Solid Edge part; units mm, degrees
sketch "Sketch1" plane through (0, 0, 0) normal (0, -1, 0) x (1, 0, 0)
  line L0 (-30, 3.5) -> (30, 3.5)
  line L1 (30, 3.5) -> (30, -3.5)
  line L2 (30, -3.5) -> (-30, -3.5)
  line L3 (-30, -3.5) -> (-30, 3.5)
  dimension "D1" = 30
  dimension "D2" = 30
extrude "Protrusion1" add sketch "Sketch1" against normal blind 70
sketch "Sketch2" plane through (0, 35, 3.5) normal (0, 0, 1) x (0, 1, 0)
  line L0 (15, 3) -> (-15, 3)
  line L1 (-15, 3) -> (-15, -3)
  line L2 (-15, -3) -> (15, -3)
  line L3 (15, -3) -> (15, 3)
  dimension "D1" = 15
  dimension "D2" = 15
extrude "Utskärning_för_vertikal_pelare" cut sketch "Sketch2" against normal blind 5
fillet "Avrundningar_1" radius 1 8 edges at (-30, 35, 3.5) (0, 0, 3.5) (30, 35, 3.5) (0, 70, 3.5) (30, 70, 0) (30, 0, 0) (-30, 70, 0) (-30, 0, 0)
Can you work these out from the model? Positions are in its coordinate system, mm. A direction names the side the tool comes from. Round coordinates to 2 decimals unless told otherwise and drop trailing zeros. Order: outer loops, then holes, each group sorted by start corner. A loop starts at its lowest first (then second) coordinate and runs counter-clockwise, first axis right, second up. Notation, with made-up numbers: (85.25, -39.5) -> (125.25, -39.5) arc R16 ccw to (125.25, -25.5) -> close; hole circle Ø2 at (-14, 2.5). An arc over 180 degrees is marked (long way). Return JSON: item names as keys, results as strings. Group by question number.
1. If we section it at B-B, the plane x = -1: Write out the boundary of the cut face in (y, z), then the cut area to 3 significant figures.
2. If we section it at A-A, the plane y = 25: Write out the boundary of the cut face in (x, z), then the cut area to 3 significant figures.
3. If we section it at C-C, the plane z = 1: Write out the boundary of the cut face in (x, y), then the cut area to 3 significant figures.
4. I need wall thicknesses on line 1 (X direction, y = 27, z = 1.25); line 2 (X direction, y = 41.5, z = 3); line 3 (X direction, y = 66, z = 3). Which ranges of each line are inside material? Lowest first, please. Write a range as [from, to].
5. We'd pull the mould along Y, two halves only. Please class faces 3 (the face through (0, 0, -1)), 4 (the face through (3, 35, 1)), 5 (the face through (0, 35, -1.5)), 6 (the face through (0, 35, -3.5)): released by +Y, released by -Y, zero draft, split by the parting line, or undercut.
6. Which directions (+Z, -Z, +X, -X, +Y, -Y) give clear straight access to the entire face, cutting with the end or side of a thin tool? Please do faces 1 (the face through (-3, 35, 1)), 2 (the face through (-30, 35, -1)).
Output values:
{
 "1": {"outline": "(0, -3.5) -> (70, -3.5) -> (70, 2.5) arc R1 ccw to (69, 3.5) -> (50, 3.5) -> (50, -1.5) -> (20, -1.5) -> (20, 3.5) -> (1, 3.5) arc R1 ccw to (0, 2.5) -> close", "area": "340 mm²"},
 "2": {"outline": "(-30, -3.5) -> (30, -3.5) -> (30, 2.5) arc R1 ccw to (29, 3.5) -> (3, 3.5) -> (3, -1.5) -> (-3, -1.5) -> (-3, 3.5) -> (-29, 3.5) arc R1 ccw to (-30, 2.5) -> close", "area": "390 mm²"},
 "3": {"outline": "(-30, 1) arc R1 ccw to (-29, 0) -> (29, 0) arc R1 ccw to (30, 1) -> (30, 69) arc R1 ccw to (29, 70) -> (-29, 70) arc R1 ccw to (-30, 69) -> close; hole (-3, 20) -> (3, 20) -> (3, 50) -> (-3, 50) -> close", "area": "4,020 mm²"},
 "4": {"line 1": "[-30, -3], [3, 30]", "line 2": "[-29.87, -3], [3, 29.87]", "line 3": "[-29.87, 29.87]"},
 "5": {"face 3": "released by -Y", "face 4": "undercut", "face 5": "undercut", "face 6": "zero draft"},
 "6": {"face 1": "+Z", "face 2": "+Z, -Z, -X, +Y, -Y"}
}
